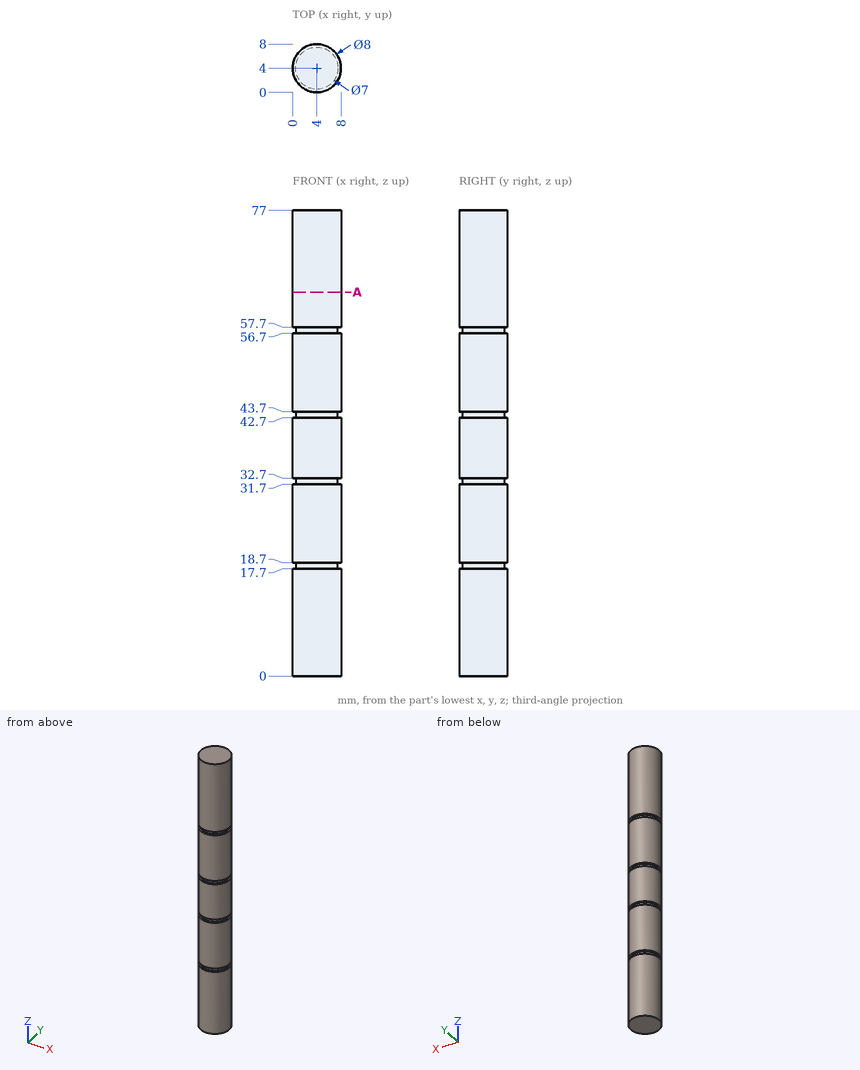
Geometry: see drawing. Coordinates: mm, zero at the bounding-box minimum. Round coordinates to 2 decimals unless told otherwise and drop trailing zeros. Loops run counter-clockwise (first coordinate to the right, second up) from the corner with the lowest first, then second, coordinate; pieces in that order, holes last. Notation, with made-up numbers: (69.25, -5.75) - (94.25, -5.75) arc R18 ccw to (94.25, 10.25) - close; hole circle Ø6 at (34.5, 79.25). An arc over 180 degrees is marked (long way). Use CSV: the item, a comma, the result in double quotes.
Q1. Pin query (flat end, axial travel): pin 1 Ø1 at (x, z) = (5.5, 22.5) entering from +Y. Return the tip coordinate at first contact, or that it passes through.
Reported:
pin 1,"y = 7.87"
Q2. Ray query, line 1 along Z through (x, y) = (0.5, 3); line 2 along X through (y, z) = (4.25, 63.5); line 3 along X through (y, z) = (2.25, 6.5). Return the intervals inside material, ascending.
Reported:
line 1,"0 to 17.7, 18.7 to 31.7, 32.7 to 42.7, 43.7 to 56.7, 57.7 to 77"
line 2,"0.01 to 7.99"
line 3,"0.4 to 7.6"
Q3. Section query A-A, the plane z = 63.5. Output: boundary loops of the cut face in (x, y), then the cut area to 3 significant figures.
Reported:
outline,"circle Ø8 at (4, 4)"
area,"50.3 mm^2"
